```python
from build123d import *

# Parameters (mm, degrees)
F0_W     = 55
F0_H     = 130
F1_DEPTH = 3
F3_R     = 1.5
F4_DEPTH = 25
F5_R     = 1.5
F6_DEPTH = 25


with BuildPart() as f1:
    # F0 (on Top) → F1 (new body)
    with BuildSketch(Plane.XY):
        with Locations((27.5, 65)):
            Rectangle(F0_W, F0_H)
    extrude(amount=F1_DEPTH)

    # F3 (on face) → F4 (cut)
    with BuildSketch(Plane.XY.offset(3)):
        with Locations((27.4549201131, 43.8495948911)):
            Circle(F3_R)
    extrude(amount=-F4_DEPTH, mode=Mode.SUBTRACT)

    # F5 (on face) → F6 (cut)
    with BuildSketch(Plane.XY.offset(3)):
        with Locations((27.5, 114.1266003251)):
            Circle(F5_R)
    extrude(amount=-F6_DEPTH, mode=Mode.SUBTRACT)

    # F8: F1 across plane


with BuildPart() as f1_1:
    add(f1.part)
    add(f1.part.mirror(Plane.YZ))


solid = f1_1.part
```
The model under review builds one solid part; all positions refer to its coordinate system, in mm. Coordinates: 2 decimals unless noted, no trailing zeros. Order: outer loops, then holes, each group sorted by start corner. A loop starts at its lowest first (then second) coordinate and runs counter-clockwise, first axis right, second up. Notation, with made-up numbers: M 56.5,-36 L 69.5,-36 A6 cw 69.5,-26 Z; hole C -22,29.25 d5. An arc over 180 degrees is marked long. One line per question, with ' | ' between items.
(1) Add section A-A, the plane x = -27.5. Write out the cut boundary in (y, z), then the cut area to 3 significant figures.
Geometry results:
outline: M 0,0 L 42.35,0 L 42.35,3 L 0,3 Z; M 45.35,0 L 112.63,0 L 112.63,3 L 45.35,3 Z; M 115.63,0 L 130,0 L 130,3 L 115.63,3 Z | area: 372 mm²
(2) Insertion check: pin 1 (1.8 mm diameter, centred on x = 27.45, y = 43.85, fed in from +Z). The pin has a flat end and moves straight along its axis. Give the tip position at first contact, or say it passes through.
Geometry results:
pin 1: passes through
(3) For probe 1 along X at (y, z) = (114, 2.45); probe 2 along Y at (x, z) = (27.5, 1.1); probe 3 along Y at (x, z) = (27, 1.55), list the stretches that pass through material, from the lowest coordinate up. Write a range as from..to.
Geometry results:
probe 1: x = -55..-28.99, -26.01..26.01, 28.99..55 | probe 2: y = 0..42.35, 45.35..112.63, 115.63..130 | probe 3: y = 0..42.42, 45.28..112.71, 115.54..130
(4) The part is to be moulded in two halves that separate along X. For faces 1 (the face through (55, 64, 1)), 2 (the face through (1, 66, 0)), 3 (the face through (-27.26, 45.337, 1.521)), say which applies: +X half, -X half, draft (parallel to the pull), parting line (faces both ways), or undercut.
Geometry results:
face 1: +X half | face 2: draft | face 3: undercut
